For this review, take the finished solid that the model builds, in its own axes (mm). A direction names the side the tool comes from. Give positions to 0.01 mm unless a question says otherwise; leave off trailing zeros. Write each loop counter-clockwise with the first axis right and the second up, starting at its lowest first coordinate (ties: lowest second). Pieces come first, ordered by that corner, then holes. Notation, with made-up numbers: (-3.5, -1.5) -> (47.5, -1.5) arc R22 cw to (47.5, 25.5) -> close; hole circle Ø4 at (31, 68.5). An arc over 180 degrees is marked (long way). Return JSON: item names as keys, results as strings.
from build123d import *

# Parameters (mm, degrees)
SKETCH1_R           = 21
SKETCH1_R_2         = 1.5
BOSS_EXTRUDE1_DEPTH = 6
CUT_EXTRUDE1_DEPTH  = 6
CIRPATTERN1_COUNT   = 40
CUT_EXTRUDE2_REACH  = 8
BOSS_EXTRUDE2_DEPTH = 6
BOSS_EXTRUDE3_DEPTH = 7
CUT_EXTRUDE4_REACH  = 15
SKETCH7_W           = 0.5
SKETCH7_H           = 20
CUT_EXTRUDE5_REACH  = 8


with BuildPart() as part:
    # Sketch1 → Boss-Extrude1 (new body)
    with BuildSketch(Plane(origin=(0, 0, 0), x_dir=(1, 0, 0), z_dir=(0, 1, 0))):
        Circle(SKETCH1_R)
        Circle(SKETCH1_R_2, mode=Mode.SUBTRACT)
    extrude(amount=BOSS_EXTRUDE1_DEPTH)

    # Sketch2 → Cut-Extrude1 (cut)
    with BuildSketch(Plane(origin=(0, 6, 0), x_dir=(1, 0, 0), z_dir=(0, 1, 0))):
        with BuildLine():
            Line((-0.870178472, 18.980062946), (-0.412307542, 20.99595205))
            ThreePointArc((-0.412307542, 20.99595205), (0, 21), (0.412307542, 20.99595205))
            Line((0.412307542, 20.99595205), (0.870178472, 18.980062946))
            ThreePointArc((0.870178472, 18.980062946), (1.180608684, 18.963284608), (1.490722819, 18.941429341))
            Line((1.490722819, 18.941429341), (1.73143755, 22))
            Line((1.73143755, 22), (-1.73143755, 22))
            Line((-1.73143755, 22), (-1.490722819, 18.941429341))
            ThreePointArc((-1.490722819, 18.941429341), (-1.180608684, 18.963284608), (-0.870178472, 18.980062946))
        make_face()
    cut_extrude1 = extrude(amount=-CUT_EXTRUDE1_DEPTH, mode=Mode.SUBTRACT)

    # CirPattern1: Cut-Extrude1 ×40 about axis
    cirpattern1_axis = Axis((0, 0, 0), (0, 1, 0))
    for i in range(1, CIRPATTERN1_COUNT):
        add(cut_extrude1.rotate(cirpattern1_axis, i * 360 / CIRPATTERN1_COUNT), mode=Mode.SUBTRACT)

    # Sketch3 → Cut-Extrude2 (cut, up to next)
    with BuildSketch(Plane(origin=(0, 6, 0), x_dir=(1, 0, 0), z_dir=(0, 1, 0)), mode=Mode.PRIVATE) as cut_extrude2_sk1:
        with BuildLine():
            Line((-4, 0), (-20.367312321, 5.115915248))
            ThreePointArc((-20.367312321, 5.115915248), (5.753143593, -20.196567501), (14.614168728, 15.080652253))
            Line((14.614168728, 15.080652253), (4, 0))
            Line((4, 0), (-4, 0))
        make_face()
    cut_extrude2_tool1 = extrude(cut_extrude2_sk1.sketch, amount=-CUT_EXTRUDE2_REACH, mode=Mode.PRIVATE) & part.part
    add(cut_extrude2_tool1.solids().sort_by_distance((1.540678, 6, 6.01351))[0], mode=Mode.SUBTRACT)

    # Sketch4 → Boss-Extrude2 (add)
    with BuildSketch(Plane.XZ):
        with BuildLine():
            Line((1.5, 0), (4, 0))
            Line((4, 0), (4, 141.5))
            ThreePointArc((4, 141.5), (3.121320344, 143.621320344), (1, 144.5))
            Line((1, 144.5), (-1, 144.5))
            ThreePointArc((-1, 144.5), (-3.121320344, 143.621320344), (-4, 141.5))
            Line((-4, 141.5), (-4, 0))
            Line((-4, 0), (-1.5, 0))
            ThreePointArc((-1.5, 0), (0, 1.5), (1.5, 0))
        make_face()
    extrude(amount=-BOSS_EXTRUDE2_DEPTH)

    # Sketch5 → Boss-Extrude3 (add)
    with BuildSketch(Plane.XZ):
        with BuildLine():
            Line((-4, 141.5), (-4, 119.5))
            Line((-4, 119.5), (0, 119.5))
            Line((0, 119.5), (0, 144.5))
            Line((0, 144.5), (-1, 144.5))
            ThreePointArc((-1, 144.5), (-3.121320344, 143.621320344), (-4, 141.5))
        make_face()
    extrude(amount=BOSS_EXTRUDE3_DEPTH)

    # Sketch7 → Cut-Extrude4 (cut, up to next)
    with BuildSketch(Plane.XZ.offset(7), mode=Mode.PRIVATE) as cut_extrude4_sk1:
        with Locations((-2, 131.5)):
            Rectangle(SKETCH7_W, SKETCH7_H)
    cut_extrude4_tool1 = extrude(cut_extrude4_sk1.sketch, amount=-CUT_EXTRUDE4_REACH, mode=Mode.PRIVATE) & part.part
    add(cut_extrude4_tool1.solids().sort_by_distance((-2, -7, 131.5))[0], mode=Mode.SUBTRACT)

    # Sketch8 → Cut-Extrude5 (cut, up to next)
    with BuildSketch(Plane.XZ, mode=Mode.PRIVATE) as cut_extrude5_sk1:
        with BuildLine():
            Line((-1.2, 10), (-1.2, 109.5))
            ThreePointArc((-1.2, 109.5), (0, 110.7), (1.2, 109.5))
            Line((1.2, 109.5), (1.2, 10))
            ThreePointArc((1.2, 10), (0, 8.8), (-1.2, 10))
        make_face()
    cut_extrude5_tool1 = extrude(cut_extrude5_sk1.sketch, amount=-CUT_EXTRUDE5_REACH, mode=Mode.PRIVATE) & part.part
    add(cut_extrude5_tool1.solids().sort_by_distance((0, 0, 59.75))[0], mode=Mode.SUBTRACT)


solid = part.part
1. For faces 1 (the flat face through (-2, -3, 119.5)), 2 (the flat face through (0, -3, 132)), 3 (the flat face through (1.2, 3, 60)), 4 (the flat face through (-4, 2, 72)), 5 (the flat face through (4, 3, 70)), list the 3-axis set-ups (+Z, -Z, +X, -X, +Y, -Y) from which the entire face can be reached by the end or side of a thin tool; tool diameter is ignored.
Results found:
{"face 1": "-Z, +X, -X, -Y", "face 2": "+Z, -Z, +X, -Y", "face 3": "+Y, -Y", "face 4": "+Z, -X, +Y, -Y", "face 5": "+Z, +X, +Y, -Y"}
2. For pin 1 (4 mm diameter, centred on y = 3, z = 79.5, fed in from -X); pin 2 (2 mm diameter, centred on x = 3, z = 63, fed in from -Y); pin 3 (3 mm diameter, centred on y = 2.5, z = 65, fed in from +X), all flat-tipped, find the tip position at first contact; note any pin that passes through.
Results found:
{"pin 1": "stops at x = -4", "pin 2": "stops at y = 0", "pin 3": "stops at x = 4"}
3. Add section A-A, the plane z = 106. State the section outline as (x, y) points, plus the area to 3 significant figures.
Results found:
{"outline": "(-4, 0) -> (-1.2, 0) -> (-1.2, 6) -> (-4, 6) -> close; (1.2, 0) -> (4, 0) -> (4, 6) -> (1.2, 6) -> close", "area": "33.6 mm²"}
4. To check wall thickness, follow probe 1 along Z at (x, y) = (0, 2); probe 2 along X at (y, z) = (5, 80.5); probe 3 along X at (y, z) = (-4, 134). State the ranges of each line that lie inside material, in increasing order.
Results found:
{"probe 1": "z = -21 to -1.5, 1.5 to 8.8, 110.7 to 144.5", "probe 2": "x = -4 to -1.2, 1.2 to 4", "probe 3": "x = -4 to -2.25, -1.75 to 0"}
5. The part is to be moulded in two halves that separate along X. For faces 6 (the cylindrical face through (3.14, 2.96, 143.6)), 7 (the flat face through (-2.25, -1, 131)), 8 (the flat face through (-2, 6, 50)), say which applies: +X half, -X half, draft (parallel to the pull), parting line (faces both ways), or undercut.
Results found:
{"face 6": "+X half", "face 7": "undercut", "face 8": "draft"}
6. Add section B-B, the plane y = -3. State the section outline as (x, z) points.
Results found:
{"outline": "(-4, 119.5) -> (0, 119.5) -> (0, 144.5) -> (-1, 144.5) arc R3 ccw to (-4, 141.5) -> close; hole (-2.25, 121.5) -> (-1.75, 121.5) -> (-1.75, 141.5) -> (-2.25, 141.5) -> close"}
7. Add section C-C, the plane z = 7. State the section outline as (x, y) points, plus the area to 3 significant figures.
Results found:
{"outline": "(-4, 0) -> (4, 0) -> (4, 6) -> (-4, 6) -> close", "area": "48.0 mm²"}
